Source: CAD feature listing. Evaluate the final solid. Frame: model axes, mm. A direction names the side the tool comes from. Give positions to 0.01 mm unless a question says otherwise; leave off trailing zeros. Order: outer loops, then holes, each group sorted by start corner. A loop starts at its lowest first (then second) coordinate and runs counter-clockwise, first axis right, second up. Notation, with made-up numbers: M 21.25,59 L 71.25,59 A15 ccw 71.25,72 Z; hole C -8.5,27 d5. An arc over 180 degrees is marked long. One line per question, with ' | ' between items. Start each with the question number.
from build123d import *

# Parameters (mm, degrees)
F2_DEPTH = 3
F3_R     = 2
F4_R     = 1


with BuildPart() as f2:
    # F1 (on Top) → F2 (new body)
    with BuildSketch(Plane.XY):
        with BuildLine():
            ThreePointArc((-6.3245553203, -3), (-7, 0), (-6.3245553203, 3))
            Line((-6.3245553203, 3), (-12.5, 3))
            Line((-12.5, 3), (-12.5, -3))
            Line((-12.5, -3), (-6.3245553203, -3))
        make_face()
        with BuildLine():
            Line((6.3245553203, -3), (2.7207535721, -3))
            ThreePointArc((2.7207535721, -3), (0, -4.05), (-2.7207535721, -3))
            Line((-2.7207535721, -3), (-6.3245553203, -3))
            ThreePointArc((-6.3245553203, -3), (0, -7), (6.3245553203, -3))
        make_face()
        with BuildLine():
            ThreePointArc((-2.7207535721, -3), (-4.05, 0), (-2.7207535721, 3))
            Line((-2.7207535721, 3), (-6.3245553203, 3))
            ThreePointArc((-6.3245553203, 3), (-7, 0), (-6.3245553203, -3))
            Line((-6.3245553203, -3), (-2.7207535721, -3))
        make_face()
        with BuildLine():
            ThreePointArc((-2.7207535721, 3), (0, 4.05), (2.7207535721, 3))
            Line((2.7207535721, 3), (6.3245553203, 3))
            ThreePointArc((6.3245553203, 3), (0, 7), (-6.3245553203, 3))
            Line((-6.3245553203, 3), (-2.7207535721, 3))
        make_face()
        with BuildLine():
            ThreePointArc((2.7207535721, 3), (3.7028065009, 1.6406474382), (4.05, 0))
            ThreePointArc((4.05, 0), (3.7028065009, -1.6406474382), (2.7207535721, -3))
            Line((2.7207535721, -3), (6.3245553203, -3))
            ThreePointArc((6.3245553203, -3), (6.8290514437, -1.5375488216), (7, 0))
            ThreePointArc((7, 0), (6.8290514437, 1.5375488216), (6.3245553203, 3))
            Line((6.3245553203, 3), (2.7207535721, 3))
        make_face()
        with BuildLine():
            Line((12.5, 3), (6.3245553203, 3))
            ThreePointArc((6.3245553203, 3), (6.8290514437, 1.5375488216), (7, 0))
            ThreePointArc((7, 0), (6.8290514437, -1.5375488216), (6.3245553203, -3))
            Line((6.3245553203, -3), (12.5, -3))
            Line((12.5, -3), (12.5, 3))
        make_face()
    extrude(amount=F2_DEPTH)

    # F3
    f3_edges = [f2.edges().sort_by_distance(p)[0] for p in [
        (-12.5, -3, 1.5),
        (-12.5, 3, 1.5),
        (12.5, -3, 1.5),
        (12.5, 3, 1.5),
    ]]
    fillet(f3_edges, radius=F3_R)

    # F4
    f4_edges = [f2.edges().sort_by_distance(p)[0] for p in [
        (-12.5, 0, 3),
        (-11.914214, 2.414214, 3),
        (-11.914214, -2.414214, 3),
        (-8.412278, 3, 3),
        (-8.412278, -3, 3),
        (0, 7, 3),
        (0, -7, 3),
        (8.412278, 3, 3),
        (8.412278, -3, 3),
        (11.914214, 2.414214, 3),
        (11.914214, -2.414214, 3),
        (12.5, 0, 3),
        (-2.720754, -3, 3),
    ]]
    fillet(f4_edges, radius=F4_R)


solid = f2.part
Item 1: Line query: line 1 (Z direction, x = -3, y = 5.25); line 2 (Y direction, x = 9.75, z = 0.2); line 3 (Y direction, x = 3.5, z = 1.7). Output: solid intervals per line, ascending.
Item 2: Cut plane B-B on x = -10.25. Return the cut outline in (y, z), and give its area (3 significant figures).
Item 3: Cut plane A-A on z = 1.4. Return the cut outline in (x, y).
Item 4: Pin query (flat end, axial travel): pin 1 Ø1 at (x, z) = (8, 1) entering from +Y; pin 2 Ø1.6 at (x, z) = (7.5, 1.5) entering from -Y. Return the tip coordinate at first contact, or that it passes through.
Item 5: Reachability of faces 1 (the flat face through (8, -3, 1)), 2 (the flat face through (-8, -3, 1)), 3 (the flat face through (8, 3, 1)), 4 (the cylindrical face through (8.112, -2.699, 2.715)), 5 (the cylindrical face through (8.045, 2.699, 2.715)) from +Z, -Z, +X, -X, +Y, -Y: full face, straight path, thin tool, end or side. Return the list, or none.
Results are:
1) line 1: z = 0 to 3 | line 2: y = -3 to 3 | line 3: y = -6.06 to -2.04, 2.04 to 6.06
2) outline: M -3,0 L 3,0 L 3,2 A1 ccw 2,3 L -2,3 A1 ccw -3,2 Z | area: 17.6 mm2
3) outline: M -12.5,-1 A2 ccw -10.5,-3 L -6.32,-3 A7 ccw 6.32,-3 L 10.5,-3 A2 ccw 12.5,-1 L 12.5,1 A2 ccw 10.5,3 L 6.32,3 A7 ccw -6.32,3 L -10.5,3 A2 ccw -12.5,1 Z; hole C 0,0 d8.1
4) pin 1: stops at y = 3 | pin 2: stops at y = -3
5) face 1: +Z, -Z, +X, -Y | face 2: +Z, -Z, -X, -Y | face 3: +Z, -Z, +X, +Y | face 4: +Z, +X, -Y | face 5: +Z, +X, +Y
